Work out the finished part from the listing and answer in its coordinate system (mm). A direction names the side the tool comes from. Round coordinates to 2 decimals unless told otherwise and drop trailing zeros. Write each loop counter-clockwise with the first axis right and the second up, starting at its lowest first coordinate (ties: lowest second). Pieces come first, ordered by that corner, then holes. Notation, with made-up numbers: (9, 43) -> (51, 43) arc R11 ccw to (51, 55) -> close; hole circle Ø3 at (-17, 9.25). An arc over 180 degrees is marked (long way). Answer as a JSON object with one key per item and string values. Group by question number.
from build123d import *

# Parameters (mm, degrees)
MAIN_SERVO_BODY_DEPTH       = 19.8
SERVO_BRACKET_DEPTH         = 30.3
SKETCH3_R                   = 6.5
SERVO_AXIS_1_DEPTH          = 2
SERVO_BRACKET_SUPPORT_DEPTH = 0.75
SKETCH5_R                   = 2.85
SERVO_AXIS_2_DEPTH          = 3
SKETCH6_R                   = 2.5
SERVO_WIRES_DEPTH           = 2
SERVO_CONTOURING_R          = 1


with BuildPart() as part:
    # Sketch1 → Main Servo Body (new body)
    with BuildSketch(Plane.XY):
        Polygon((0, 0), (40.6, 0), (40.6, 26.8), (47, 26.8), (47, 29.3), (40.6, 29.3), (40.6, 33.6), (37.6, 36.6), (3, 36.6), (0, 33.6), (0, 29.3), (-6.4, 29.3), (-6.4, 26.8), (0, 26.8), align=None)
    extrude(amount=MAIN_SERVO_BODY_DEPTH)

    # Sketch2 → Servo Bracket (cut, through all)
    with BuildSketch(Plane(origin=(0, 29.3, 0), x_dir=(1, 0, 0), z_dir=(0, 1, 0))):
        with BuildLine():
            Line((-6.4, -3.7), (-4.8, -3.7))
            ThreePointArc((-4.8, -3.7), (-2.4, -4.9), (-4.8, -6.1))
            Line((-4.8, -6.1), (-6.4, -6.1))
            Line((-6.4, -6.1), (-6.4, -3.7))
        make_face()
        with BuildLine():
            Line((45.4, -3.7), (47, -3.7))
            Line((47, -3.7), (47, -6.1))
            Line((47, -6.1), (45.4, -6.1))
            ThreePointArc((45.4, -6.1), (43, -4.9), (45.4, -3.7))
        make_face()
        with BuildLine():
            Line((45.4, -13.7), (47, -13.7))
            Line((47, -13.7), (47, -16.1))
            Line((47, -16.1), (45.4, -16.1))
            ThreePointArc((45.4, -16.1), (43, -14.9), (45.4, -13.7))
        make_face()
        with BuildLine():
            Line((-6.4, -16.1), (-6.4, -13.7))
            Line((-6.4, -13.7), (-4.8, -13.7))
            ThreePointArc((-4.8, -13.7), (-2.4, -14.9), (-4.8, -16.1))
            Line((-4.8, -16.1), (-6.4, -16.1))
        make_face()
    extrude(amount=-SERVO_BRACKET_DEPTH, mode=Mode.SUBTRACT)

    # Sketch3 → Servo Axis 1 (add)
    with BuildSketch(Plane(origin=(0, 36.6, 0), x_dir=(1, 0, 0), z_dir=(0, 1, 0))):
        with Locations((10, -10.1)):
            Circle(SKETCH3_R)
    extrude(amount=SERVO_AXIS_1_DEPTH)

    # Sketch4 → Servo Bracket Support (add, symmetric)
    with BuildSketch(Plane.XY.offset(10.1)):
        Polygon((-5.5, 29.3), (0, 31.3), (0, 29.3), align=None)
        Polygon((40.6, 29.3), (46.1, 29.3), (40.6, 31.3), align=None)
    extrude(amount=SERVO_BRACKET_SUPPORT_DEPTH, both=True)

    # Sketch5 → Servo Axis 2 (add)
    with BuildSketch(Plane(origin=(0, 38.6, 0), x_dir=(1, 0, 0), z_dir=(0, 1, 0))):
        with Locations((10, -10.1)):
            Circle(SKETCH5_R)
    extrude(amount=SERVO_AXIS_2_DEPTH)

    # Sketch6 → Servo Wires (add)
    with BuildSketch(Plane.ZY):
        with Locations((10.1, 6)):
            Circle(SKETCH6_R)
    extrude(amount=SERVO_WIRES_DEPTH)

    # Servo Contouring
    servo_contouring_edges = [part.edges().sort_by_distance(p)[0] for p in [
        (40.6, 13.4, 19.8),
        (3.5, 38.6, 10.1),
        (-6.4, 28.05, 0),
        (0, 31.45, 0),
        (40.6, 31.45, 0),
        (47, 28.05, 19.8),
        (47, 28.05, 0),
        (40.6, 13.4, 0),
        (20.3, 0, 0),
        (0, 13.4, 0),
        (40.6, 31.45, 19.8),
        (40.6, 0, 9.9),
        (0, 0, 9.9),
        (0, 31.45, 19.8),
        (0, 13.4, 19.8),
        (-6.4, 28.05, 19.8),
        (20.3, 0, 19.8),
    ]]
    fillet(servo_contouring_edges, radius=SERVO_CONTOURING_R)


solid = part.part
1) A cutting plane is placed at B-B on x = -1. Determine the outline of the cut face in (y, z), plus the area to 3 significant figures.
2) A cutting plane is placed at C-C on z = 2.5. Determine the outline of the cut face in (x, y).
3) For a pull along Y with two mould halves and no side action, classify faces 5 (the face through (43.388, 30.286, 10.11)), 6 (the face through (-0.99, 7.69, 8.26)), 7 (the face through (43, 28.1, 14.9)) as released by +Y, released by -Y, zero draft, split by the parting line, or undercut.
4) Straight lines are drawn through the part: L1, parallel to Z at x = -3, y = 27; L2, parallel to Z at x = 44.5, y = 28.6; L3, parallel to X at y = 9.5, z = 8.75. For each, find the intervals that lie inside material, in ascending order.
5) A cutting plane is placed at A-A on y = 7.5. Determine the outline of the cut face in (x, z).
6) A cutting plane is placed at D-D on x = 33.5. Determine the outline of the cut face in (y, z).
7) A tool of negligible diameter and unlimited length cuts with its end or side. For faces 1 (the face through (7.738, 40.079, 11.834)), 2 (the face through (-1, 30, 10.85)), 3 (the face through (46, 28, 16.1)), 4 (the face through (-1, 30, 9.35)), from which of +Z, -Z, +X, -X, +Y, -Y can it reach the whole face along a straight path? Write none if from no direction.
8) Each of these flat-tipped pins is pushed along its axis until it touches: P1, Ø1.5, axis at x = 27.5, z = 12.5, coming from the +Y side; P2, Ø2.5, axis at x = -3.9, z = 14.9, coming from the -Y side; P3, Ø8, axis at x = 44, z = 7, coming from the -Y side; P4, Ø9, axis at y = 15.5, z = 12.5, coming from the +X side. Where does it stop, or does it pass through?
Established:
{
 "1": {"outline": "circle Ø5 at (6, 10.1); (26.8, 0) -> (29.3, 0) -> (29.3, 9.35) -> (30.94, 9.35) -> (30.94, 10.85) -> (29.3, 10.85) -> (29.3, 19.8) -> (26.8, 19.8) -> close", "area": "71.6 mm²"},
 "2": {"outline": "(-6.4, 26.8) -> (0, 26.8) -> (0, 1) arc R1 ccw to (1, 0) -> (39.6, 0) arc R1 ccw to (40.6, 1) -> (40.6, 26.8) -> (47, 26.8) -> (47, 29.3) -> (40.6, 29.3) -> (40.6, 33.6) -> (37.6, 36.6) -> (3, 36.6) -> (0, 33.6) -> (0, 29.3) -> (-6.4, 29.3) -> close"},
 "3": {"face 5": "released by +Y", "face 6": "undercut", "face 7": "zero draft"},
 "4": {"L1": "z = 0 to 3.7, 6.1 to 13.7, 16.1 to 19.8", "L2": "z = 0 to 3.4, 6.4 to 13.4, 16.4 to 19.8", "L3": "x = 0 to 40.6"},
 "5": {"outline": "(-2, 8.1) -> (0, 8.1) -> (0, 1) arc R1 ccw to (1, 0) -> (39.6, 0) arc R1 ccw to (40.6, 1) -> (40.6, 18.8) arc R1 ccw to (39.6, 19.8) -> (1, 19.8) arc R1 ccw to (0, 18.8) -> (0, 12.1) -> (-2, 12.1) -> close"},
 "6": {"outline": "(0, 1) arc R1 ccw to (1, 0) -> (36.6, 0) -> (36.6, 19.8) -> (1, 19.8) arc R1 ccw to (0, 18.8) -> close"},
 "7": {"face 1": "+Y", "face 2": "+Z, -X, +Y", "face 3": "+X, +Y, -Y", "face 4": "-Z, -X, +Y"},
 "8": {"P1": "stops at y = 36.6", "P2": "passes through", "P3": "stops at y = 0.08", "P4": "stops at x = 40.6"}
}
